Design review of the part built by this model. Coordinates are the model's own, in mm. Face numbers are marked on the shaded views. A direction names the side the tool comes from. Give positions to 0.01 mm unless a question says otherwise; leave off trailing zeros. Order: outer loops, then holes, each group sorted by start corner. A loop starts at its lowest first (then second) coordinate and runs counter-clockwise, first axis right, second up. Notation, with made-up numbers: (21, -7.75) -> (46, -7.75) arc R18 cw to (46, 9.25) -> close; hole circle Ø8 at (69, 23). An arc over 180 degrees is marked (long way). Return JSON: item names as keys, results as strings.
Autodesk Inventor part; units mm, degrees
ref_plane "YZ Plane" through (0, 0, 0) normal (1, 0, 0) x (0, 1, 0)
ref_plane "XZ Plane" through (0, 0, 0) normal (0, 1, 0) x (-1, 0, 0)
ref_plane "XY Plane" through (0, 0, 0) normal (0, 0, 1) x (1, 0, 0)
sketch "Sketch1" plane through (0, 0, 0) normal (0, 1, 0) x (-1, 0, 0)
  line L0 (0, 0) -> (21.1582, 0)
  line L1 (21.1582, 0) -> (21.1582, 16.3576)
  line L2 (21.1582, 16.3576) -> (0, 16.3576)
  line L3 (0, 16.3576) -> (0, 0)
  dimension "d0" = 21.1582
  dimension "d1" = 16.3576
extrude "Extrusion1" add sketch "Sketch1" along normal blind 1.4478
sketch "Sketch2" plane through (0, 1.4478, 0) normal (0, 1, 0) x (1, 0, 0)
  line L0 (0, 0) -> (-21.1582, 0)
  line L1 (-21.1582, 0) -> (-21.1582, -16.3576)
  line L2 (0, -16.3576) -> (0, 0)
  circle A0 centre (-18.8468, -2.3114) radius 1.651
  circle A1 centre (-2.3114, -2.3114) radius 1.651
  dimension "d4" = 0.6604
  dimension "d5" = 0.6604
  dimension "d6" = 0.6604
  dimension "d7" = 3.302
extrude "Extrusion2" cut sketch "Sketch2" against normal through all
sketch "Sketch3" plane through (0, 1.4478, 0) normal (0, 1, 0) x (1, 0, 0)
  line L0 (0, 0) -> (-21.1582, 0)
  line L1 (-12.1539, -2.286) -> (-9.0043, -2.286)
  line L2 (-9.0043, -2.286) -> (-9.0043, -3.8735)
  line L3 (-9.0043, -3.8735) -> (-12.1539, -3.8735)
  line L4 (-12.1539, -3.8735) -> (-12.1539, -2.286)
  point P0 (-10.5791, -2.286)
  point P1 (-10.5791, 0)
  dimension "d10" = 3.1496
  dimension "d11" = 1.5875
  dimension "d12" = 2.286
extrude "Extrusion3" add sketch "Sketch3" along normal blind 1.8161
sketch "Sketch4" plane through (0, 1.4478, 0) normal (0, 1, 0) x (1, 0, 0)
  line L0 (-9.0043, -3.8735) -> (-12.1539, -3.8735)
  line L1 (0, 0) -> (-21.1582, 0)
  line L2 (-8.6741, -5.3086) -> (-12.4841, -5.3086)
  line L3 (-12.4841, -5.3086) -> (-12.4841, -9.1186)
  line L4 (-12.4841, -9.1186) -> (-8.6741, -9.1186)
  line L5 (-8.6741, -9.1186) -> (-8.6741, -5.3086)
  line L6 (-8.6741, -5.3086) -> (-12.4841, -9.1186) construction
  line L7 (-12.4841, -5.3086) -> (-8.6741, -9.1186) construction
  point P0 (-10.5791, -7.2136)
  point P1 (-10.5791, 0)
  point P2 (-10.5791, -7.2136)
  dimension "d15" = 3.81
  dimension "d16" = 3.81
  dimension "d17" = 1.4351
extrude "Extrusion4" add sketch "Sketch4" along normal blind 0.762
sketch "Sketch5" plane through (0, 1.4478, 0) normal (0, 1, 0) x (1, 0, 0)
  line L0 (-21.1582, 0) -> (-21.1582, -16.3576)
  line L1 (-21.1582, -16.3576) -> (0, -16.3576)
  circle A0 centre (-19.3662, -14.5656) radius 0.776
  dimension "d20" = 1.016
  dimension "d21" = 1.016
extrude "Extrusion5" cut sketch "Sketch5" against normal through all
sketch "Sketch6" plane through (0, 1.4478, 0) normal (0, 1, 0) x (1, 0, 0)
  circle A0 centre (-19.3662, -14.5656) radius 0.776
  circle A1 centre (-19.3662, -14.5656) radius 0.889
  dimension "d24" = 1.778
extrude "Extrusion6" add sketch "Sketch6" along normal blind 0.0254
pattern_linear "Rectangular Pattern1" count 8 spacing 2.54 along (1, 0, 0) of "Extrusion5", "Extrusion6"
equation "\"d5\" = d4"
equation "\"d6\" = d5"
properties part number "GY-521 Gyro"
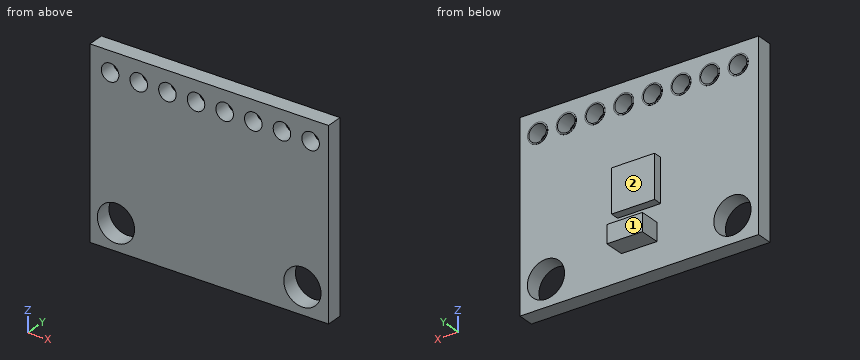
Item 1: Add section C-C (z = 1.5). Give the boundary of the cut face in (x, y), plus the area to 3 significant figures.
Result set:
{"outline": "(-21.16, 0) -> (-20.28, 0) -> (-20.28, 1.45) -> (-21.16, 1.45) -> close; (-17.41, 0) -> (-3.75, 0) -> (-3.75, 1.45) -> (-17.41, 1.45) -> close; (-0.87, 0) -> (0, 0) -> (0, 1.45) -> (-0.87, 1.45) -> close", "area": "22.3 mm^2"}
Item 2: Add section A-A (y = 1.8). Give the boundary of the cut face in (x, z), plus the area to 3 significant figures.
Result set:
{"outline": "(-12.48, 5.31) -> (-8.67, 5.31) -> (-8.67, 9.12) -> (-12.48, 9.12) -> close; (-12.15, 2.29) -> (-9, 2.29) -> (-9, 3.87) -> (-12.15, 3.87) -> close", "area": "19.5 mm^2"}
Item 3: Machinability: for the marked faces 1 and 2, which of the approach directions +Z, -Z, +X, -X, +Y, -Y give a long, thin tool a straight path to every point of the face, cutting with its end or side? Answer none if there is none.
Result set:
{"face 1": "+Z, -Z, +X, -X, +Y", "face 2": "+Z, +X, -X, +Y"}
Item 4: For pin 1 (2 mm diameter, centred on x = -9.5, z = 14.5, fed in from +Y); pin 2 (0.5 mm diameter, centred on x = -10.5, y = 2, fed in from +Z), all flat-tipped, find the tip position at first contact; note any pin that passes through.
Result set:
{"pin 1": "stops at y = 1.47", "pin 2": "stops at z = 9.12"}
Item 5: Wall thickness on L1, parallel to Z at x = -3.5, y = 0.3; L2, parallel to Z at x = -10, y = 2.15; L3, parallel to X at y = 1.85, z = 9: over which ranges is each line inside the solid? List them lowest first. Write a range as [from, to].
Result set:
{"L1": "z = [0, 1.17], [3.46, 14.11], [15.02, 16.36]", "L2": "z = [2.29, 3.87], [5.31, 9.12]", "L3": "x = [-12.48, -8.67]"}
Item 6: Add section B-B (x = -18). Give the boundary of the cut face in (y, z), plus the area to 3 significant figures.
Result set:
{"outline": "(0, 0) -> (1.45, 0) -> (1.45, 0.89) -> (0, 0.89) -> close; (0, 3.73) -> (1.45, 3.73) -> (1.45, 16.36) -> (0, 16.36) -> close", "area": "19.6 mm^2"}
Item 7: Add section D-D (z = 7.75). Give the boundary of the cut face in (x, y).
Result set:
{"outline": "(-21.16, 0) -> (0, 0) -> (0, 1.45) -> (-8.67, 1.45) -> (-8.67, 2.21) -> (-12.48, 2.21) -> (-12.48, 1.45) -> (-21.16, 1.45) -> close"}
